```python
from build123d import *

# Parameters (mm, degrees)
SKETCH5_W                                      = 53
SKETCH5_H                                      = 37
BOSS_EXTRUDE3_DEPTH                            = 3
BOSS_EXTRUDE4_DEPTH                            = 19
BOSS_EXTRUDE4_DEPTH_BACK                       = 3
SKETCH6_W                                      = 3
SKETCH6_H                                      = 37
SKETCH7_W                                      = 7
SKETCH7_H                                      = 18.5
BOSS_EXTRUDE5_DEPTH                            = 5
FILLET3_R                                      = 3
SKETCH8_W                                      = 59
SKETCH8_H                                      = 22
SKETCH8_R                                      = 0.5
BOSS_EXTRUDE6_DEPTH                            = 2
CSK_FOR_M3_FLAT_HEAD_MACHINE_SCREW1_AT_2_COUNT = 2
CSK_FOR_M3_FLAT_HEAD_MACHINE_SCREW1_AT_2_PITCH = 42.6
BOSS_EXTRUDE7_DEPTH                            = 1.44
SKETCH11_W                                     = 18
SKETCH11_H                                     = 8.25
CUT_EXTRUDE1_DEPTH                             = 3.5
SKETCH12_W                                     = 18
SKETCH12_H                                     = 8.25
CUT_EXTRUDE2_DEPTH                             = 3.5


with BuildPart() as part:
    # Sketch5 → Boss-Extrude3 (new body)
    with BuildSketch(Plane.XY):
        with Locations((26.5, 18.5)):
            Rectangle(SKETCH5_W, SKETCH5_H)
    extrude(amount=BOSS_EXTRUDE3_DEPTH)

    # Sketch6 → Boss-Extrude4 (add, two sides: drawn at the far end of the back side and taken through both)
    with BuildSketch(Plane.XY.offset(3).offset(-BOSS_EXTRUDE4_DEPTH_BACK)):
        with Locations((-1.5, 18.5)):
            Rectangle(SKETCH6_W, SKETCH6_H)
        with Locations((54.5, 18.5)):
            Rectangle(SKETCH6_W, SKETCH6_H)
    extrude(amount=BOSS_EXTRUDE4_DEPTH + BOSS_EXTRUDE4_DEPTH_BACK)

    # Sketch7 → Boss-Extrude5 (add)
    # profile 1 of 2: a face of its own
    with BuildSketch(Plane.XY.offset(22)):
        with Locations((-6.5, 18.5)):
            Rectangle(SKETCH7_W, SKETCH7_H)
        with BuildLine():
            Line((-6, 25.25), (-6, 11.75))
            ThreePointArc((-6, 11.75), (-6.5, 11.25), (-7, 11.75))
            Line((-7, 11.75), (-7, 25.25))
            ThreePointArc((-7, 25.25), (-6.5, 25.75), (-6, 25.25))
        make_face(mode=Mode.SUBTRACT)
    # profile 2 of 2: a face of its own
    with BuildSketch(Plane.XY.offset(22)):
        with Locations((59.5, 18.5)):
            Rectangle(SKETCH7_W, SKETCH7_H)
        with BuildLine():
            Line((59, 25.25), (59, 11.75))
            ThreePointArc((59, 11.75), (59.5, 11.25), (60, 11.75))
            Line((60, 11.75), (60, 25.25))
            ThreePointArc((60, 25.25), (59.5, 25.75), (59, 25.25))
        make_face(mode=Mode.SUBTRACT)
    extrude(amount=-BOSS_EXTRUDE5_DEPTH)

    # Fillet3
    fillet3_edges = [part.edges().sort_by_distance(p)[0] for p in [
        (-3, 27.75, 19.5),
        (-3, 9.25, 19.5),
        (-10, 9.25, 19.5),
        (-10, 27.75, 19.5),
        (63, 9.25, 19.5),
        (56, 9.25, 19.5),
        (56, 27.75, 19.5),
        (63, 27.75, 19.5),
    ]]
    fillet(fillet3_edges, radius=FILLET3_R)

    # Sketch8 → Boss-Extrude6 (add)
    with BuildSketch(Plane.XZ):
        with Locations((26.5, 11)):
            Rectangle(SKETCH8_W, SKETCH8_H)
        with Locations((5.2, 9.5)):
            Circle(SKETCH8_R, mode=Mode.SUBTRACT)
        with Locations((47.8, 9.5)):
            Circle(SKETCH8_R, mode=Mode.SUBTRACT)
    extrude(amount=BOSS_EXTRUDE6_DEPTH)

    # Sketch9 → CSK for M3 Flat Head Machine Screw1 (revolve, cut)
    with BuildSketch(Plane(origin=(5.2, 0, 9.5), x_dir=(0, 0, 1), z_dir=(1, 0, 0))):
        Polygon((0, 0), (0, 2), (1.7, 2), (1.7, 1.45), (3.15, 0), align=None)
    csk_for_m3_flat_head_machine_screw1 = revolve(axis=Axis((5.2, 6.35, 9.5), (0, -1, 0)), mode=Mode.SUBTRACT)

    # CSK for M3 Flat Head Machine Screw1 at 2: CSK for M3 Flat Head Machine Screw1 ×2
    with Locations(*[(i * CSK_FOR_M3_FLAT_HEAD_MACHINE_SCREW1_AT_2_PITCH, 0, 0) for i in range(1, CSK_FOR_M3_FLAT_HEAD_MACHINE_SCREW1_AT_2_COUNT)]):
        add(csk_for_m3_flat_head_machine_screw1, mode=Mode.SUBTRACT)

    # Sketch10 → Boss-Extrude7 (add)
    with BuildSketch(Plane(origin=(0, 37, 0), x_dir=(1, 0, 0), z_dir=(0, 1, 0))):
        Polygon((0, -22), (-3, -22), (-3, 0), (56, 0), (56, -22), (53, -22), (53, -3), (0, -3), align=None)
    extrude(amount=BOSS_EXTRUDE7_DEPTH)

    # Sketch11 → Cut-Extrude1 (cut)
    with BuildSketch(Plane.ZY.offset(3)):
        with Locations((13, 2.125)):
            Rectangle(SKETCH11_W, SKETCH11_H)
    extrude(amount=-CUT_EXTRUDE1_DEPTH, mode=Mode.SUBTRACT)

    # Sketch12 → Cut-Extrude2 (cut)
    with BuildSketch(Plane(origin=(56, 0, 0), x_dir=(0, 0, -1), z_dir=(1, 0, 0))):
        with Locations((-13, 2.125)):
            Rectangle(SKETCH12_W, SKETCH12_H)
    extrude(amount=-CUT_EXTRUDE2_DEPTH, mode=Mode.SUBTRACT)


solid = part.part
```
The listing builds one solid part. Answer for the finished solid, in the listing's coordinates (mm). A direction names the side the tool comes from. Give positions to 0.01 mm unless a question says otherwise; leave off trailing zeros. Order: outer loops, then holes, each group sorted by start corner. A loop starts at its lowest first (then second) coordinate and runs counter-clockwise, first axis right, second up.
1) Find section A-A on y = 19. Write down the section's boundary in (x, z).
Reported:
outline: (-10, 17) - (-7, 17) - (-7, 22) - (-10, 22) - close; (-6, 17) - (-3, 17) - (-3, 0) - (56, 0) - (56, 17) - (59, 17) - (59, 22) - (53, 22) - (53, 3) - (0, 3) - (0, 22) - (-6, 22) - close; (60, 17) - (63, 17) - (63, 22) - (60, 22) - close
2) Given P1, Ø10, axis at y = 10, z = 3, coming from the +X side; P2, Ø1.6, axis at y = -1.5, z = 11.5, coming from the +X side; P3, Ø3.5, axis at x = -8, y = 14, coming from the -Z side; P4, Ø8, axis at x = 32, y = 11.5, coming from the -Z side, each flat-ended and moving along its own axis, determine where each tip first touches the part or whether it passes through.
Reported:
P1: stops at x = 56
P2: stops at x = 52.5
P3: stops at z = 17
P4: stops at z = 0
3) Find section D-D on x = 35. Write down the section's boundary in (y, z), then the cut area to 3 significant figures.
Reported:
outline: (-2, 0) - (38.44, 0) - (38.44, 3) - (0, 3) - (0, 22) - (-2, 22) - close
area: 159 mm2
4) For faces 1 (the face through (-5.8, 18.7, 17)), 2 (the face through (55, 6.25, 13)), 3 (the face through (60, 18, 20)), determine the directions among +Z, -Z, +X, -X, +Y, -Y from which every point of the face is accessible in a straight line to the end or side of a thin tool.
Reported:
face 1: -Z, -X, +Y, -Y
face 2: +Z, +X, -X, -Y
face 3: +Z, -Z
5) Find section C-C on x = 5.2. Write down the section's boundary in (y, z), then the cut area to 3 significant figures.
Reported:
outline: (-2, 0) - (38.44, 0) - (38.44, 3) - (0, 3) - (0, 6.35) - (-1.45, 7.8) - (-2, 7.8) - close; (-2, 11.2) - (-1.45, 11.2) - (0, 12.65) - (0, 22) - (-2, 22) - close
area: 150 mm2
6) Determine the mould class of faces 4 (the face through (49.46, -1.72, 9.13)), 5 (the face through (6.23, -1.72, 8.15)), 6 (the face through (0.5, -1, 13)), 7 (the face through (54, 2, 4)) for opening direction Z: pulls with the +Z half, pulls with the -Z half, needs draft (parallel to the pull), parting line crosses it, or undercut.
Reported:
face 4: undercut
face 5: undercut
face 6: needs draft
face 7: pulls with the +Z half
7) Find section B-B on z = 9.5. Write down the section's boundary in (x, y), then the cut area to 3 significant figures.
Reported:
outline: (-3, 6.25) - (0, 6.25) - (0, 38.44) - (-3, 38.44) - close; (0.5, -2) - (3.5, -2) - (3.5, -1.45) - (2.05, 0) - (0.5, 0) - close; (6.9, -2) - (46.1, -2) - (46.1, -1.45) - (44.65, 0) - (8.35, 0) - (6.9, -1.45) - close; (49.5, -2) - (52.5, -2) - (52.5, 0) - (50.95, 0) - (49.5, -1.45) - close; (53, 6.25) - (56, 6.25) - (56, 38.44) - (53, 38.44) - close
area: 279 mm2
8) Consider line 1 along X through (y, z) = (-1.6, 9.5); line 2 along X through (y, z) = (34, 10); line 3 along Z through (x, y) = (5.2, -1.6). Determine where each line is inside the solid, lowest interval first.
Reported:
line 1: x = 0.5 to 3.5, 6.9 to 46.1, 49.5 to 52.5
line 2: x = -3 to 0, 53 to 56
line 3: z = 0 to 7.8, 11.2 to 22
